Verification items for the finished model (mm, model axes). Face numbers are marked on the shaded views. Coordinates: 2 decimals unless noted, no trailing zeros. Loops run counter-clockwise (first coordinate to the right, second up) from the corner with the lowest first, then second, coordinate; pieces in that order, holes last.
Q1. Sectioned sample at C-C (z = 151). Enter the section's corners in (x, y), then the cut area to 3 significant figures.
Q2. Sectioned sample at D-D (y = -15). Enter the section's corners in (x, z).
Q3. Sectioned sample at B-B (x = 0). Enter the section's corners in (y, z), then the cut area to 3 significant figures.
Q4. Material ranges on probe 1 along X at (y, z) = (13, 115); probe 2 along Y at (x, z) = (6.5, 14.5); probe 3 along X at (y, z) = (15, -56.5), recorded low to high.
Q5. Go/stop test with flat-tipped pins: P1, Ø1.5, axis at x = 9, z = -66.5, coming from the +Y side; P2, Ø1.5, axis at y = 6.5, z = 145, coming from the +X side; P3, Ø1.5, axis at x = 7.5, z = 102.5, coming from the +Y side; P4, Ø12, axis at x = -8.5, y = 11.5, coming from the -Z side. Record where each tip stops, or that it passes through.
Q6. Mould release check, pull along X, two halves, no side actions. Record for the marked faces 1 and 2: +X half, -X half, draft (parallel to the pull), parting line (faces both ways), or undercut.
Q7. Sectioned sample at A-A (y = 0). Enter the section's corners in (x, z).
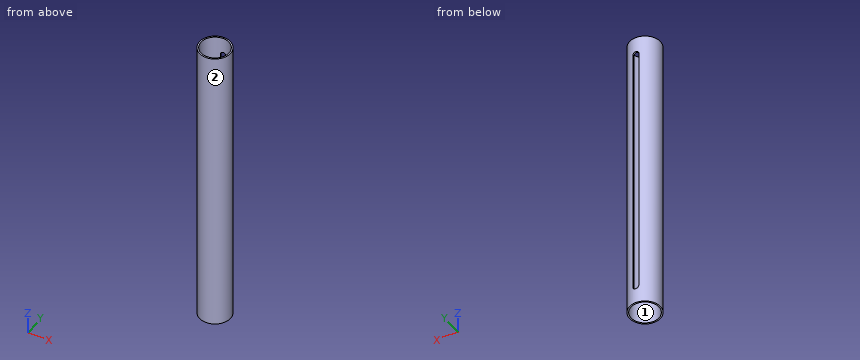
```python
from build123d import *

# Parameters (mm, degrees)
SKETCH1_R           = 21
SKETCH1_R_2         = 19
BOSS_EXTRUDE1_DEPTH = 200
CUT_EXTRUDE1_REACH  = 45


with BuildPart() as part:
    # Sketch1 → Boss-Extrude1 (new body, symmetric)
    with BuildSketch(Plane.XY):
        Circle(SKETCH1_R)
        Circle(SKETCH1_R_2, mode=Mode.SUBTRACT)
    extrude(amount=BOSS_EXTRUDE1_DEPTH, both=True)

    # Sketch2 → Cut-Extrude1 (cut, up to next)
    with BuildSketch(Plane(origin=(0, 22, 0), x_dir=(1, 0, 0), z_dir=(0, 1, 0)), mode=Mode.PRIVATE) as cut_extrude1_sk1:
        with BuildLine():
            Line((-4, -175), (-4, 175))
            ThreePointArc((-4, 175), (0, 179), (4, 175))
            Line((4, 175), (4, -175))
            ThreePointArc((4, -175), (0, -179), (-4, -175))
        make_face()
    cut_extrude1_tool1 = extrude(cut_extrude1_sk1.sketch, amount=-CUT_EXTRUDE1_REACH, mode=Mode.PRIVATE) & part.part
    add(cut_extrude1_tool1.solids().sort_by_distance((0, 22, 0))[0], mode=Mode.SUBTRACT)


solid = part.part
```
Geometry check:
1. outline: (-4, 18.57) - (-4, 20.62) arc R21 ccw (long way) to (4, 20.62) - (4, 18.57) arc R19 cw (long way) to start
1. area: 235 mm2
2. outline: (-14.7, -200) - (-11.66, -200) - (-11.66, 200) - (-14.7, 200) - close; (11.66, -200) - (14.7, -200) - (14.7, 200) - (11.66, 200) - close
3. outline: (-21, -200) - (-19, -200) - (-19, 200) - (-21, 200) - close; (19, -200) - (21, -200) - (21, -179) - (19, -179) - close; (19, 179) - (21, 179) - (21, 200) - (19, 200) - close
3. area: 884 mm2
4. probe 1: x = -16.49 to -13.86, 13.86 to 16.49
4. probe 2: y = -19.97 to -17.85, 17.85 to 19.97
4. probe 3: x = -14.7 to -11.66, 11.66 to 14.7
5. P1: stops at y = 19.31
5. P2: stops at x = 20.2
5. P3: stops at y = 19.89
5. P4: stops at z = -200
6. face 1: undercut
6. face 2: parting line
7. outline: (-21, -200) - (-19, -200) - (-19, 200) - (-21, 200) - close; (19, -200) - (21, -200) - (21, 200) - (19, 200) - close
